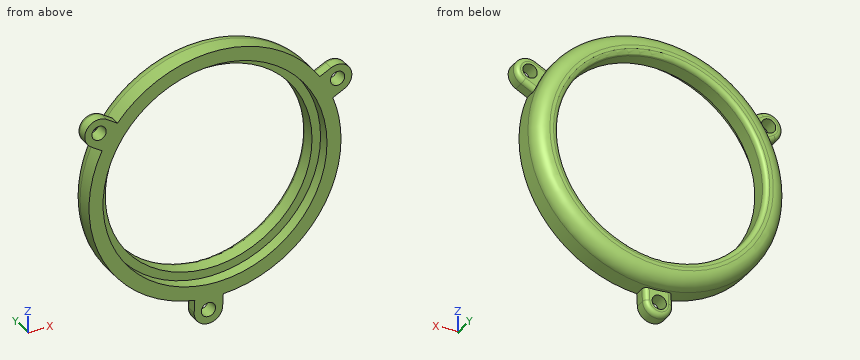
from build123d import *

# Parameters (mm, degrees)
SKETCH1_R           = 26.5
SKETCH1_R_2         = 21.75
BOSS_EXTRUDE1_DEPTH = 6.5
FILLET1_R           = 3
SKETCH2_R           = 23.55
SKETCH2_R_2         = 21.75
CUT_EXTRUDE1_DEPTH  = 2.51
SKETCH3_R           = 1.5
BOSS_EXTRUDE2_DEPTH = 3
CIRPATTERN1_COUNT   = 3
FILLET2_R           = 1
FILLET4_R           = 1


with BuildPart() as part:
    # Sketch1 → Boss-Extrude1 (new body)
    with BuildSketch(Plane(origin=(0, 0, 0), x_dir=(1, 0, 0), z_dir=(0, 1, 0))):
        Circle(SKETCH1_R)
        Circle(SKETCH1_R_2, mode=Mode.SUBTRACT)
    extrude(amount=BOSS_EXTRUDE1_DEPTH)

    # Fillet1
    fillet1_edges = [part.edges().sort_by_distance(p)[0] for p in [
        (-26.5, 6.5, 0),
    ]]
    fillet(fillet1_edges, radius=FILLET1_R)

    # Sketch2 → Cut-Extrude1 (cut)
    with BuildSketch(Plane.XZ):
        Circle(SKETCH2_R)
        Circle(SKETCH2_R_2, mode=Mode.SUBTRACT)
    extrude(amount=-CUT_EXTRUDE1_DEPTH, mode=Mode.SUBTRACT)

    # Sketch3 → Boss-Extrude2 (add)
    with BuildSketch(Plane.XZ):
        with BuildLine():
            Line((-20.523964569, 16.763558046), (-23.769018949, 11.716814337))
            Line((-23.769018949, 11.716814337), (-26.015121786, 13.161057649))
            ThreePointArc((-26.015121786, 13.161057649), (-26.915966451, 17.306956694), (-22.770067406, 18.207801359))
            Line((-22.770067406, 18.207801359), (-20.523964569, 16.763558046))
        make_face()
        with Locations((-24.392594596, 15.684429504)):
            Circle(SKETCH3_R, mode=Mode.SUBTRACT)
    boss_extrude2 = extrude(amount=-BOSS_EXTRUDE2_DEPTH)

    # CirPattern1: Boss-Extrude2 ×3 about axis
    cirpattern1_axis = Axis((0, 0, 0), (0, 1, 0))
    for i in range(1, CIRPATTERN1_COUNT):
        add(boss_extrude2.rotate(cirpattern1_axis, i * 360 / CIRPATTERN1_COUNT))

    # Fillet2
    fillet2_edges = [part.edges().sort_by_distance(p)[0] for p in [
        (-21.75, 6.5, 0),
    ]]
    fillet(fillet2_edges, radius=FILLET2_R)

    # Fillet4
    fillet4_edges = [part.edges().sort_by_distance(p)[0] for p in [
        (-21.647015988, 3, 17.485679702),
        (-24.892070368, 3, 12.438935993),
        (-26.915966451, 3, 17.306956694),
        (-4.319534831, 3, -27.489705613),
        (1.673600618, 3, -27.776633288),
        (-1.530280933, 3, -31.963389061),
        (25.966550819, 3, 10.00402591),
        (23.21846975, 3, 15.337697295),
        (28.446247385, 3, 14.656432367),
    ]]
    fillet(fillet4_edges, radius=FILLET4_R)


solid = part.part
Can you work these out from the model? Positions are in its coordinate system, mm. Coordinates: 2 decimals unless noted, no trailing zeros. Write each loop counter-clockwise with the first axis right and the second up, starting at its lowest first coordinate (ties: lowest second). Pieces come first, ordered by that corner, then holes. Notation, with made-up numbers: (88, 87.5) -> (128, 87.5) arc R20 cw to (128, 103.5) -> close; hole circle Ø11 at (-20, 3.5). An arc over 180 degrees is marked (long way). Write each question's results on one line, items separated by ' | '. Start each with the question number.
Item 1: If we section it at B-B, the plane y = 1.25: Write out the boundary of the cut face in (x, z), and give its area (3 significant figures).
Item 2: If we section it at A-A, the plane z = 0: Write out the boundary of the cut face in (x, y).
Item 3: I'm going to push flat-ended pins straight in: P1, Ø2, axis at x = 10, y = 3.5, coming from the -Z side; P2, Ø2.5, axis at x = -24.39, z = 15.68, coming from the +Y side; P3, Ø1.5, axis at y = 1, z = 17, coming from the -X side; P4, Ø1.5, axis at x = 7.5, y = 5, coming from the +Z side. Where does each tip first touch, or does it pass through?
Item 4: Please list where these lines run through material, in increasing order: probe 1 along Z at (x, y) = (-2.5, 1.25); probe 2 along Z at (x, y) = (-5, 3); probe 3 along X at (y, z) = (4, 11.5).
Answer block:
1) outline: (-26.02, 13.16) -> (-23.77, 11.72) arc R26.5 ccw to (-4.26, -26.16) -> (-4.38, -28.82) arc R3 ccw to (1.61, -29.11) -> (1.74, -26.44) arc R26.5 ccw to (24.78, 9.39) -> (27.15, 10.62) arc R3 ccw to (24.41, 15.95) -> (22.03, 14.73) arc R26.5 ccw to (-20.52, 16.76) -> (-22.77, 18.21) arc R3 ccw to start; hole circle Ø3 at (-24.39, 15.68); hole circle Ø47.1 at (0, 0); hole circle Ø3 at (-1.39, -28.97); hole circle Ø3 at (25.78, 13.28) | area: 531 mm²
2) outline: (-26.5, 0) -> (-23.55, 0) -> (-23.55, 2.51) -> (-21.75, 2.51) -> (-21.75, 5.5) arc R1 ccw to (-22.75, 6.5) -> (-23.5, 6.5) arc R3 ccw to (-26.5, 3.5) -> close; (21.75, 2.51) -> (23.55, 2.51) -> (23.55, 0) -> (26.5, 0) -> (26.5, 3.5) arc R3 ccw to (23.5, 6.5) -> (22.75, 6.5) arc R1 ccw to (21.75, 5.5) -> close
3) P1: z = -24.92 | P2: through | P3: x = -27.34 | P4: z = 25.4
4) probe 1: -31.75 to -29.97, -27.96 to -23.42, 23.42 to 26.38 | probe 2: -26.02 to -21.17, 21.17 to 26.02 | probe 3: -23.83 to -18.46, 18.46 to 23.83
